```python
from build123d import *

# Parameters (mm, degrees)
SKETCH1_W           = 140
SKETCH1_H           = 55
BOSS_EXTRUDE1_DEPTH = 2.4
SKETCH2_R           = 3
BOSS_EXTRUDE2_DEPTH = 2.6
SKETCH3_R           = 1.25
BOSS_EXTRUDE3_DEPTH = 2.5
SKETCH4_R           = 2.5
BOSS_EXTRUDE4_DEPTH = 20
SKETCH5_R           = 0.8
BOSS_EXTRUDE5_DEPTH = 2.4


with BuildPart() as part:
    # Sketch1 → Boss-Extrude1 (new body)
    with BuildSketch(Plane(origin=(0, 0, 0), x_dir=(1, 0, 0), z_dir=(0, 1, 0))):
        Rectangle(SKETCH1_W, SKETCH1_H)
    extrude(amount=BOSS_EXTRUDE1_DEPTH)

    # Sketch2 → Boss-Extrude2 (add)
    with BuildSketch(Plane(origin=(0, 2.4, 0), x_dir=(1, 0, 0), z_dir=(0, 1, 0))):
        with Locations(Location((66.5, -24.3, 0), (0, 0, 90))):
            Circle(SKETCH2_R)
        with Locations(Location((63.94, 11.65, 0), (0, 0, 90))):
            Circle(SKETCH2_R)
        with Locations(Location((22, -24.3, 0), (0, 0, 90))):
            Circle(SKETCH2_R)
        with Locations(Location((24.56, 11.65, 0), (0, 0, 90))):
            Circle(SKETCH2_R)
    extrude(amount=BOSS_EXTRUDE2_DEPTH)

    # Sketch3 → Boss-Extrude3 (add)
    with BuildSketch(Plane(origin=(0, 5, 0), x_dir=(1, 0, 0), z_dir=(0, 1, 0))):
        with Locations(Location((22, -24.3, 0), (0, 0, 270))):
            Circle(SKETCH3_R)
        with Locations(Location((24.56, 11.65, 0), (0, 0, 270))):
            Circle(SKETCH3_R)
        with Locations(Location((66.5, -24.3, 0), (0, 0, 270))):
            Circle(SKETCH3_R)
        with Locations(Location((63.94, 11.65, 0), (0, 0, 270))):
            Circle(SKETCH3_R)
    extrude(amount=BOSS_EXTRUDE3_DEPTH)

    # Sketch4 → Boss-Extrude4 (add)
    with BuildSketch(Plane(origin=(0, 2.4, 0), x_dir=(1, 0, 0), z_dir=(0, 1, 0))):
        with Locations(Location((9.56, 17.5, 0), (0, 0, 90))):
            Circle(SKETCH4_R)
        with Locations(Location((-54.44, 17.5, 0), (0, 0, 90))):
            Circle(SKETCH4_R)
        with Locations(Location((-54.44, -8.3, 0), (0, 0, 90))):
            Circle(SKETCH4_R)
        with Locations(Location((9.56, -8.3, 0), (0, 0, 90))):
            Circle(SKETCH4_R)
    extrude(amount=BOSS_EXTRUDE4_DEPTH)

    # Sketch5 → Boss-Extrude5 (add)
    with BuildSketch(Plane(origin=(0, 22.4, 0), x_dir=(1, 0, 0), z_dir=(0, 1, 0))):
        with Locations(Location((9.56, -8.3, 0), (0, 0, 270))):
            Circle(SKETCH5_R)
        with Locations(Location((9.56, 17.5, 0), (0, 0, 270))):
            Circle(SKETCH5_R)
        with Locations(Location((-54.44, 17.5, 0), (0, 0, 270))):
            Circle(SKETCH5_R)
        with Locations(Location((-54.44, -8.3, 0), (0, 0, 270))):
            Circle(SKETCH5_R)
    extrude(amount=BOSS_EXTRUDE5_DEPTH)


solid = part.part
```
Geometry check sheet. Reference: the model listing, model coordinates, mm. A direction names the side the tool comes from. Coordinates: 2 decimals unless noted, no trailing zeros. Order: outer loops, then holes, each group sorted by start corner. A loop starts at its lowest first (then second) coordinate and runs counter-clockwise, first axis right, second up. Notation, with made-up numbers: (63, 16) - (114, 16) arc R25 cw to (114, 39) - close; hole circle Ø3 at (86, 37.5). An arc over 180 degrees is marked (long way). Answer in a Markdown table with one row per item. Add a question column.
1. Section check C-C (x = 37.5). Enter the section's corners in (y, z), plus the area to 3 significant figures.
2. Section check B-B (z = 24.3). Enter the section's corners in (x, y), plus the area to 3 significant figures.
3. Section check A-A (y = 20). Enter the section's corners in (x, z).
4. Material ranges on L1, parallel to Y at x = -42, z = -11.5; L2, parallel to X at y = 6.25, z = -17; L3, parallel to X at y = 12.75, z = 10, recorded low to high. Write a range as [from, to].
5. Draft check along Z on faces 3 (the face through (-70, 1, 0)), 4 (the face through (11, 22.4, 8)), 5 (the face through (-1, 1, -27.5)). Enter one of: +Z half, -Z half, draft (parallel to the pull), parting line (faces both ways), or undercut.
6. Gauge pin test, flat ends, axial feed: pin 1 Ø4 at (x, z) = (1, 15) entering from +Y; pin 2 Ø6.5 at (x, z) = (65.5, 24) entering from +Y; pin 3 Ø8 at (y, z) = (16, 14) entering from +X. Record the tip position at first contact, or that the pin passes through.
7. Access from +Z, -Z, +X, -X, +Y, -Y to the whole of each face (thin tool, end or side, straight path). Record for faces 1 (the face through (67.74, 6.23, 24.14)), 2 (the face through (25, 7.5, -12)).
Data:
| question | item | result |
|---|---|---|
| 1 | outline | (0, -27.5) - (2.4, -27.5) - (2.4, 27.5) - (0, 27.5) - close |
| 1 | area | 132 mm² |
| 2 | outline | (-70, 0) - (70, 0) - (70, 2.4) - (69.5, 2.4) - (69.5, 5) - (67.75, 5) - (67.75, 7.5) - (65.25, 7.5) - (65.25, 5) - (63.5, 5) - (63.5, 2.4) - (25, 2.4) - (25, 5) - (23.25, 5) - (23.25, 7.5) - (20.75, 7.5) - (20.75, 5) - (19, 5) - (19, 2.4) - (-70, 2.4) - close |
| 2 | area | 380 mm² |
| 3 | outline | circle Ø5 at (-54.44, -17.5); circle Ø5 at (-54.44, 8.3); circle Ø5 at (9.56, -17.5); circle Ø5 at (9.56, 8.3) |
| 4 | L1 | y = [0, 2.4] |
| 4 | L2 | x = [-56.89, -51.99], [7.11, 12.01] |
| 4 | L3 | x = [-56.27, -52.61], [7.73, 11.39] |
| 5 | face 3 | draft |
| 5 | face 4 | undercut |
| 5 | face 5 | -Z half |
| 6 | pin 1 | stops at y = 2.4 |
| 6 | pin 2 | stops at y = 7.5 |
| 6 | pin 3 | stops at x = 11.39 |
| 7 | face 1 | +Y |
| 7 | face 2 | +Z, -Z, +X, -X, +Y |
